Here's how the part is built. I have some questions about the finished solid (model axes, mm). Face numbers are marked on the shaded views. A direction names the side the tool comes from. Round coordinates to 2 decimals unless told otherwise and drop trailing zeros. Loops run counter-clockwise (first coordinate to the right, second up) from the corner with the lowest first, then second, coordinate; pieces in that order, holes last. Notation, with made-up numbers: M -18.5,44 L 24.5,44 A29 cw 24.5,66 Z; hole C -38,42.25 d6. An arc over 180 degrees is marked long. Answer as a JSON object with one key per item and string values.
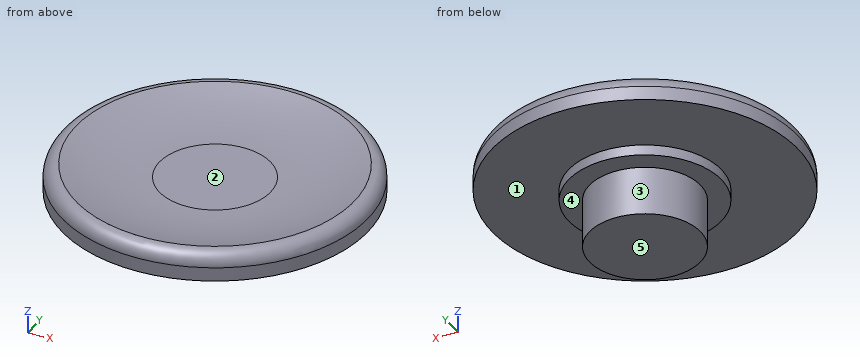
from build123d import *


with BuildPart() as f1:
    # F0 (on Front) → F1 (revolve)
    with BuildSketch(Plane.XZ):
        with BuildLine():
            Line((0, 5.25), (0, 0))
            Line((0, 0), (4, 0))
            Line((4, 0), (4, 3.5))
            Line((4, 3.5), (5.5, 3.5))
            Line((5.5, 3.5), (5.5, 4.25))
            Line((5.5, 4.25), (11, 4.25))
            Line((11, 4.25), (11, 5.25))
            ThreePointArc((11, 5.25), (10.707107, 5.957107), (10, 6.25))
            ThreePointArc((10, 6.25), (7.041381, 5.501712), (4, 5.25))
            Line((4, 5.25), (0, 5.25))
        make_face()
    revolve(axis=Axis((0, 0, 2.625), (0, 0, 1)))


solid = f1.part
Item 1: I want a section at A-A, the plane z = 1. Please give me the cut outline in (x, y).
Resolved:
{"outline": "C 0,0 d8"}
Item 2: Please list where these lines run through material, in increasing order: probe 1 along Z at (x, y) = (-4, 1.5); probe 2 along Z at (x, y) = (1.25, 3.5); probe 3 along X at (y, z) = (1.75, 1). Write a range as from..to.
Resolved:
{"probe 1": "3.5..5.25", "probe 2": "0..5.25", "probe 3": "-3.6..3.6"}
Item 3: On a 3-axis mill with a long thin cutter (end or side, diameter ignored), from which of +Z, -Z, +X, -X, +Y, -Y can I reach the whole of each face in a straight line? I mean the marked faces 4 and 5. Say none if no direction works.
Resolved:
{"face 4": "-Z", "face 5": "-Z, +X, -X, +Y, -Y"}
Item 4: If we mould it in two halves opening along Z, with no side actions, what happens to the marked faces 1, 2 and 3? For each: pulls with the +Z half, pulls with the -Z half, needs draft (parallel to the pull), parting line crosses it, or undercut.
Resolved:
{"face 1": "pulls with the -Z half", "face 2": "pulls with the +Z half", "face 3": "needs draft"}
Item 5: I'm going to push flat-ended pins straight in: pin 1 Ø4 at (x, y) = (-6.5, 0) entering from -Z; pin 2 Ø4 at (x, y) = (-7, -8.5) entering from -Z; pin 3 Ø9 at (x, y) = (-1.5, 1.5) entering from +Z. Where does each tip first touch, or does it pass through?
Resolved:
{"pin 1": "z = 3.5", "pin 2": "z = 4.25", "pin 3": "z = 5.44"}
